For this review, take the finished solid that the model builds, in its own axes (mm). A direction names the side the tool comes from. Coordinates: 2 decimals unless noted, no trailing zeros. Write each loop counter-clockwise with the first axis right and the second up, starting at its lowest first coordinate (ties: lowest second). Pieces come first, ordered by that corner, then holes.
```python
from build123d import *


with BuildPart() as f1:
    # F0 (on Front) → F1 (revolve)
    with BuildSketch(Plane.XZ):
        with BuildLine():
            Line((4.075, 0), (0, 0))
            Line((0, 0), (0, -57.4416))
            Line((0, -57.4416), (4.950736, -57.4416))
            ThreePointArc((4.950736, -57.4416), (5.014312, -57.434786), (5.075, -57.414654))
            ThreePointArc((5.075, -57.414654), (5.12167, -57.388139), (5.162868, -57.353732))
            Line((5.162868, -57.353732), (5.5166, -57))
            Line((5.5166, -57), (5.5166, -55))
            Line((5.5166, -55), (5.275, -55))
            ThreePointArc((5.275, -55), (5.133579, -54.941421), (5.075, -54.8))
            Line((5.075, -54.8), (5.075, -50))
            Line((5.075, -50), (4.075, -50))
            Line((4.075, -50), (4.075, 0))
        make_face()
    revolve(axis=Axis((0, 0, -28.7208), (0, 0, -1)))


solid = f1.part
```
Q1. Clearance check with flat-ended pins moving along their axes: pin 1 Ø1 at (y, z) = (-1.5, -23) entering from -X; pin 2 Ø6 at (x, y) = (-1, 3) entering from +Z; pin 3 Ø4 at (y, z) = (4, -41.5) entering from -X; pin 4 Ø3 at (x, z) = (-3, -6) entering from +Y. State where each tip first meets the part, or that it passes through.
Ans:
pin 1: stops at x = -3.95
pin 2: stops at z = 0
pin 3: stops at x = -3.55
pin 4: stops at y = 3.79
Q2. Add section D-D (z = -50.5). State the section outline as (x, y) points (3 decimals).
Ans:
outline: circle Ø10.15 at (0, 0)
Q3. For probe 1 along Z at (x, y) = (-1, 4); probe 2 along X at (y, z) = (-0.25, -11); probe 3 along Y at (x, z) = (3.5, -11), list the stretches that pass through material, from the lowest coordinate up.
Ans:
probe 1: z = -57.44 to -50
probe 2: x = -4.07 to 4.07
probe 3: y = -2.09 to 2.09
Q4. Add section A-A (x = 0). State the section outline as (y, z) points (3 decimals).
Ans:
outline: (-5.517, -57) - (-5.163, -57.354) arc R0.3 ccw to (-5.075, -57.415) arc R0.3 ccw to (-4.951, -57.442) - (4.951, -57.442) arc R0.3 ccw to (5.075, -57.415) arc R0.3 ccw to (5.163, -57.354) - (5.517, -57) - (5.517, -55) - (5.275, -55) arc R0.2 cw to (5.075, -54.8) - (5.075, -50) - (4.075, -50) - (4.075, 0) - (-4.075, 0) - (-4.075, -50) - (-5.075, -50) - (-5.075, -54.8) arc R0.2 cw to (-5.275, -55) - (-5.517, -55) - close
Q5. Tool access review of faces 1 (the flat face through (0, 0, 0)), 2 (the cylindrical face through (-4.027, 3.088, -52.366)): name each direction out of +Z, -Z, +X, -X, +Y, -Y from which nothing blocks a thin tool from reaching the whole face with its end or side.
Ans:
face 1: +Z, +X, -X, +Y, -Y
face 2: +Z
Q6. Add section C-C (z = -40.5). State the section outline as (x, y) points (3 decimals), then the cut area to 3 significant figures.
Ans:
outline: circle Ø8.15 at (0, 0)
area: 52.2 mm2
